Part model, mm, in its own coordinate system. Round coordinates to 2 decimals unless told otherwise and drop trailing zeros. Loops run counter-clockwise (first coordinate to the right, second up) from the corner with the lowest first, then second, coordinate; pieces in that order, holes last. Notation, with made-up numbers: M 55,45 L 82,45 A27 ccw 82,81 Z; hole C 11,75 d5. An arc over 180 degrees is marked long. Put each result on its own line as item: value. Start each with the question number.
1) Drop a flat-ended pin along its axis: pin 1 Ø2 at (y, z) = (21, 4) entering from -X. Give the stop position or say it passes through.
2) Probe line 1 along X through (y, z) = (24, 0.3); line 2 along X through (y, z) = (23.5, 0.85); line 3 along X through (y, z) = (27.25, 3.75). List the from-to ranges inside material, lowest first.
3) Slice it at B-B on y = 29.5. Give the cut face in (x, z), then the cut area to 3 significant figures.
4) Slice it at C-C on x = -71. Give the cut face in (y, z).
5) Slice it at A-A on z = 3.45. Give the cut face in (x, y), then the cut area to 3 significant figures.
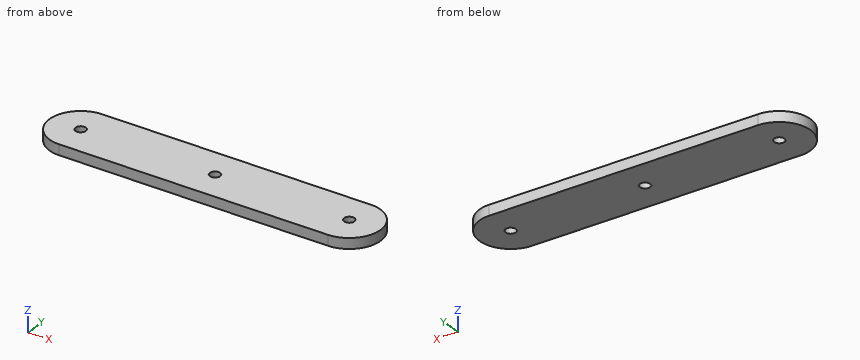
```python
from build123d import *

# Parameters (mm, degrees)
SKETCH1_R           = 2.5
BOSS_EXTRUDE1_DEPTH = 5
SKETCH2_R           = 2.5
CUT_EXTRUDE1_DEPTH  = 5


with BuildPart() as part:
    # Sketch1 → Boss-Extrude1 (new body)
    with BuildSketch(Plane.XY):
        with BuildLine():
            Line((-67.024818312, 37.285306338), (62.975181688, 37.285306338))
            ThreePointArc((62.975181688, 37.285306338), (77.975181688, 22.285306338), (62.975181688, 7.285306338))
            Line((62.975181688, 7.285306338), (-67.024818312, 7.285306338))
            ThreePointArc((-67.024818312, 7.285306338), (-82.024818312, 22.285306338), (-67.024818312, 37.285306338))
        make_face()
        with Locations((-67.024818312, 22.285306338)):
            Circle(SKETCH1_R, mode=Mode.SUBTRACT)
        with Locations((62.975181688, 22.285306338)):
            Circle(SKETCH1_R, mode=Mode.SUBTRACT)
    extrude(amount=BOSS_EXTRUDE1_DEPTH)

    # Sketch2 → Cut-Extrude1 (cut)
    with BuildSketch(Plane(origin=(0, 0, 0), x_dir=(-1, 0, 0), z_dir=(0, 0, -1))):
        with Locations((2.024818312, 22.285306338)):
            Circle(SKETCH2_R)
    extrude(amount=-CUT_EXTRUDE1_DEPTH, mode=Mode.SUBTRACT)


solid = part.part
```
Recorded:
1. pin 1: stops at x = -82.02
2. line 1: x = -81.93 to -68.84, -65.21 to -3.84, -0.21 to 61.16, 64.79 to 77.88
2. line 2: x = -81.98 to -69.21, -64.84 to -4.21, 0.16 to 60.79, 65.16 to 77.93
2. line 3: x = -81.18 to 77.13
3. outline: M -80.18,0 L 76.13,0 L 76.13,5 L -80.18,5 Z
3. area: 782 mm2
4. outline: M 7.82,0 L 36.75,0 L 36.75,5 L 7.82,5 Z
5. outline: M -67.02,7.29 L 62.98,7.29 A15 ccw 62.98,37.29 L -67.02,37.29 A15 ccw Z; hole C -67.02,22.29 d5; hole C -2.02,22.29 d5; hole C 62.98,22.29 d5
5. area: 4,550 mm2
